```python
from build123d import *

# Parameters (mm, degrees)
F1_DEPTH = 2
F3_D     = 3
F5_D     = 3


with BuildPart() as f1:
    # F0 (on Right) → F1 (new body)
    with BuildSketch(Plane.YZ):
        with BuildLine():
            Line((42.4517345428, 32.4551947415), (-31.2479986618, 32.4551947415))
            ThreePointArc((-31.2479986618, 32.4551947415), (-33.0066323151, 32.1357083536), (-34.540522163, 31.2180778109))
            Line((-34.540522163, 31.2180778109), (-42.1629837432, 24.5484222763))
            ThreePointArc((-42.1629837432, 24.5484222763), (-43.4236249385, 22.8516203396), (-43.870460242, 20.7855392069))
            Line((-43.870460242, 20.7855392069), (-43.870460242, 13.2886583044))
            ThreePointArc((-43.870460242, 13.2886583044), (-42.1023347006, 9.4735583733), (-38.0484652484, 8.3566886947))
            Line((-38.0484652484, 8.3566886947), (43.2737295365, 21.9103887931))
            ThreePointArc((43.2737295365, 21.9103887931), (46.2668344739, 23.6104839442), (47.4517345428, 26.8423584027))
            Line((47.4517345428, 26.8423584027), (47.4517345428, 27.4551947415))
            ThreePointArc((47.4517345428, 27.4551947415), (45.9872684488, 30.9907286474), (42.4517345428, 32.4551947415))
        make_face()
    extrude(amount=F1_DEPTH)

    # F3 (through all)
    with Locations(Plane(origin=(0, 0, 0), x_dir=(0, 1, 0), z_dir=(-1, 0, 0))):
        with Locations((41.4517345428, -27.4551947415), (16.4517345428, -27.4551947415)):
            Hole(F3_D / 2)

    # F5 (through all)
    with Locations(Plane(origin=(0, 0, 0), x_dir=(0, 1, 0), z_dir=(-1, 0, 0))):
        with Locations((-31.5209182738, -27.4626488093), (-38.870460242, -13.2886583044)):
            Hole(F5_D / 2)


solid = f1.part
```
Design review of the part built by this model. Coordinates are the model's own, in mm. Coordinates: 2 decimals unless noted, no trailing zeros. Order: outer loops, then holes, each group sorted by start corner. A loop starts at its lowest first (then second) coordinate and runs counter-clockwise, first axis right, second up. Notation, with made-up numbers: (-32.5, 65) -> (2.5, 65) arc R19 cw to (2.5, 90) -> close; hole circle Ø11 at (-1, 16). An arc over 180 degrees is marked (long way). One line per item, written item: value. Start each with the question number.
Q1. Take a section at B-B, the plane y = -10. State the section outline as (x, z) points, then the cut area to 3 significant figures.
Q2. Mouldability with a two-part tool opening along Y and no side actions: class faces 1 (the cylindrical face through (1.01, 16.65, 25.97)), 2 (the flat face through (1, -43.87, 17)), 3 (the cylindrical face through (0.99, 46.23, 23.57)) as pulls with the +Y half, pulls with the -Y half, needs draft (parallel to the pull), parting line crosses it, or undercut.
Q3. Take a section at C-C, the plane z = 23.5. State the section outline as (x, y) points, then the cut area to 3 significant figures.
Q4. Insertion check: pin 1 Ø2.5 at (y, z) = (16.45, 27.46) entering from +X. The pin has a flat end and moves straight along its axis. Give the tip position at first contact, or say it passes through.
Q5. Take a section at A-A, the plane x = 1.45. State the section outline as (y, z) points, then the cut area to 3 significant figures.
Q6. For probe 1 along Y at (x, z) = (1.5, 26.5); probe 2 along Y at (x, z) = (1.1, 28.75); probe 3 along Y at (x, z) = (1.1, 25), list the stretches that pass through material, from the lowest coordinate up.
Values follow:
1. outline: (0, 13.03) -> (2, 13.03) -> (2, 32.46) -> (0, 32.46) -> close
1. area: 38.8 mm2
2. face 1: undercut
2. face 2: pulls with the -Y half
2. face 3: pulls with the +Y half
3. outline: (0, -43.07) -> (2, -43.07) -> (2, 46.17) -> (0, 46.17) -> close
3. area: 178 mm2
4. pin 1: passes through
5. outline: (-43.87, 13.29) arc R5 ccw to (-38.05, 8.36) -> (43.27, 21.91) arc R5 ccw to (47.45, 26.84) -> (47.45, 27.46) arc R5 ccw to (42.45, 32.46) -> (-31.25, 32.46) arc R5 ccw to (-34.54, 31.22) -> (-42.16, 24.55) arc R5 ccw to (-43.87, 20.79) -> close; hole circle Ø3 at (-38.87, 13.29); hole circle Ø3 at (-31.52, 27.46); hole circle Ø3 at (16.45, 27.46); hole circle Ø3 at (41.45, 27.46)
5. area: 1,500 mm2
6. probe 1: y = -39.93 to -32.67, -30.37 to 15.3, 17.61 to 40.3, 42.61 to 47.44
6. probe 2: y = -37.36 to -32.29, -30.75 to 15.69, 17.21 to 40.69, 42.21 to 47.28
6. probe 3: y = -41.65 to 47.1
